The model under review builds one solid part; all positions refer to its coordinate system, in mm. Face numbers are marked on the shaded views. A direction names the side the tool comes from. Round coordinates to 2 decimals unless told otherwise and drop trailing zeros. Order: outer loops, then holes, each group sorted by start corner. A loop starts at its lowest first (then second) coordinate and runs counter-clockwise, first axis right, second up. Notation, with made-up numbers: M 68,-12 L 109,-12 A23 cw 109,15 Z; hole C -28,50.5 d9. An arc over 180 degrees is marked long. Answer as a JSON object with one key per item and string values. Group by question number.
1. Add section A-A on y = 0. State the section outline as (x, z) points (3 decimals), and give its area (3 significant figures).
2. Machinability: for the marked faces 3, 4 and 5, which of the approach directions +Z, -Z, +X, -X, +Y, -Y give a long, thin tool a straight path to every point of the face, cutting with its end or side? Answer none if there is none.
3. Mouldability with a two-part tool opening along Y and no side actions: class the marked faces 1 and 2 as released by +Y, released by -Y, zero draft, split by the parting line, or undercut.
4. Add section D-D on y = 1.7. State the section outline as (x, z) points, and give its area (3 significant figures).
5. To check wall thickness, follow probe 1 along Z at (x, y) = (1.25, 0.85); probe 2 along Z at (x, y) = (0.3, 0.7); probe 3 along X at (y, z) = (-1.9, 8.5). State the ranges of each line that lie inside material, in increasing order. Write a range as [from, to].
6. Add section B-B on x = -2. State the section outline as (y, z) points.
```python
from build123d import *

# Parameters (mm, degrees)
F0_R     = 2.286
F1_DEPTH = 10.16
F2_R     = 1.27
F3_DEPTH = 1.27
F4_R     = 2.286
F5_DEPTH = 1.27
F6_R     = 0.635
F7_DEPTH = 2.54


with BuildPart() as f1:
    # F0 (on Top) → F1 (new body)
    with BuildSketch(Plane.XY):
        Circle(F0_R)
    extrude(amount=F1_DEPTH)

    # F2 (on face) → F3 (join)
    with BuildSketch(Plane.XY.offset(10.16)):
        Circle(F2_R)
    extrude(amount=F3_DEPTH)

    # F4 (on face) → F5 (join)
    with BuildSketch(Plane.XY.offset(11.43)):
        Circle(F4_R)
    extrude(amount=F5_DEPTH)

    # F6 (on face) → F7 (join)
    with BuildSketch(Plane(origin=(0, 0, 0), x_dir=(1, 0, 0), z_dir=(0, 0, -1))):
        Circle(F6_R)
    extrude(amount=F7_DEPTH)


solid = f1.part
```
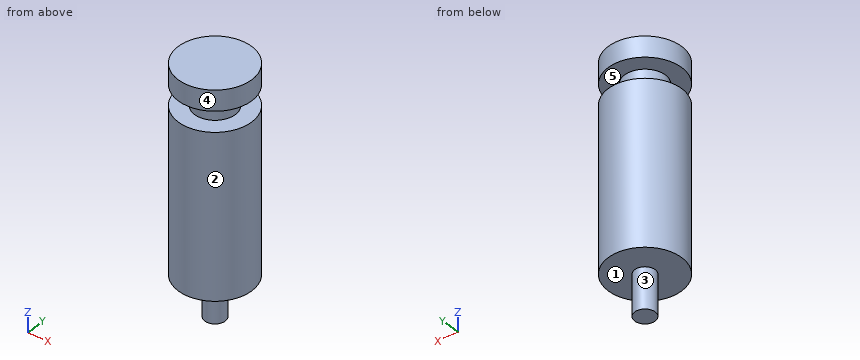
Recorded:
{
 "1": {"outline": "M -2.286,0 L -0.635,0 L -0.635,-2.54 L 0.635,-2.54 L 0.635,0 L 2.286,0 L 2.286,10.16 L 1.27,10.16 L 1.27,11.43 L 2.286,11.43 L 2.286,12.7 L -2.286,12.7 L -2.286,11.43 L -1.27,11.43 L -1.27,10.16 L -2.286,10.16 Z", "area": "58.7 mm²"},
 "2": {"face 3": "-Z", "face 4": "+Z, -Z", "face 5": "none"},
 "3": {"face 1": "zero draft", "face 2": "split by the parting line"},
 "4": {"outline": "M -1.53,0 L 1.53,0 L 1.53,10.16 L -1.53,10.16 Z; M -1.53,11.43 L 1.53,11.43 L 1.53,12.7 L -1.53,12.7 Z", "area": "34.9 mm²"},
 "5": {"probe 1": "z = [0, 10.16], [11.43, 12.7]", "probe 2": "z = [0, 12.7]", "probe 3": "x = [-1.27, 1.27]"},
 "6": {"outline": "M -1.11,0 L 1.11,0 L 1.11,10.16 L -1.11,10.16 Z; M -1.11,11.43 L 1.11,11.43 L 1.11,12.7 L -1.11,12.7 Z"}
}
